Geometry check sheet. Reference: the model listing, model coordinates, mm. Give positions to 0.01 mm unless a question says otherwise; leave off trailing zeros. Write each loop counter-clockwise with the first axis right and the second up, starting at its lowest first coordinate (ties: lowest second). Pieces come first, ordered by that corner, then holes. Notation, with made-up numbers: (73.25, 23.25) - (111.25, 23.25) arc R13 ccw to (111.25, 35.25) - close; hole circle Ø10 at (13, 48.5). An arc over 180 degrees is marked (long way). Use a Markdown table: item, result.
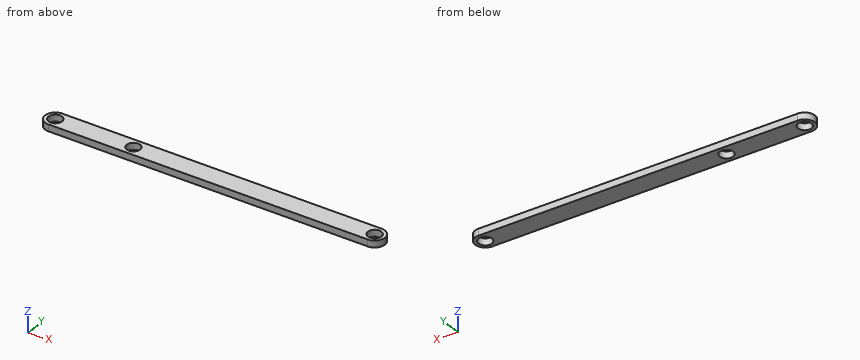
```python
from build123d import *

# Parameters (mm, degrees)
SKETCH3_W           = 250
SKETCH3_H           = 15
BOSS_EXTRUDE4_DEPTH = 5
SKETCH7_R           = 5
CUT_EXTRUDE3_DEPTH  = 5
SKETCH8_R           = 5
CUT_EXTRUDE5_DEPTH  = 6


with BuildPart() as part:
    # Sketch3 → Boss-Extrude4 (new body)
    with BuildSketch(Plane.XY):
        with Locations((-125, 7.5)):
            Rectangle(SKETCH3_W, SKETCH3_H)
    extrude(amount=BOSS_EXTRUDE4_DEPTH)

    # Sketch7 → Cut-Extrude3 (cut)
    with BuildSketch(Plane.XY.offset(5)):
        with BuildLine():
            Line((-242.499999991, 15), (-250, 15))
            Line((-250, 15), (-250, 7.5))
            ThreePointArc((-250, 7.5), (-247.803300856, 12.803300862), (-242.499999991, 15))
        make_face()
        with Locations((-242.5, 7.5)):
            Circle(SKETCH7_R)
        with BuildLine():
            ThreePointArc((-242.5, 0), (-247.803300859, 2.196699141), (-250, 7.5))
            Line((-250, 7.5), (-250, 0))
            Line((-250, 0), (-242.5, 0))
        make_face()
        with BuildLine():
            ThreePointArc((0, 7.5), (-2.196699166, 2.196699116), (-7.50000007, 0))
            Line((-7.50000007, 0), (0, 0))
            Line((0, 0), (0, 7.5))
        make_face()
        with BuildLine():
            Line((0, 15), (-7.5, 15))
            ThreePointArc((-7.5, 15), (-2.196699141, 12.803300859), (0, 7.5))
            Line((0, 7.5), (0, 15))
        make_face()
        with Locations((-7.5, 7.5)):
            Circle(SKETCH7_R)
    extrude(amount=-CUT_EXTRUDE3_DEPTH, mode=Mode.SUBTRACT)

    # Sketch8 → Cut-Extrude5 (cut, through all)
    with BuildSketch(Plane.XY.offset(5)):
        with Locations((-185, 7.5)):
            Circle(SKETCH8_R)
    extrude(amount=-CUT_EXTRUDE5_DEPTH, mode=Mode.SUBTRACT)


solid = part.part
```
1) Section check C-C on x = -185. Record the boundary of the cut face in (y, z), then the cut area to 3 significant figures.
Working result:
| item | result |
|---|---|
| outline | (0, 0) - (2.5, 0) - (2.5, 5) - (0, 5) - close; (12.5, 0) - (15, 0) - (15, 5) - (12.5, 5) - close |
| area | 25.0 mm² |
2) Depth check by flat-ended pin: P1, Ø3, axis at y = 10.5, z = 4.5, coming from the +X side; P2, Ø2, axis at y = 5, z = 1, coming from the -X side; P3, Ø3, axis at y = 1.5, z = 1.5, coming from the +X side. Enter the tip coordinate at first touch or a pass-through.
Working result:
| item | result |
|---|---|
| P1 | stops at x = -0.15 |
| P2 | stops at x = -249.85 |
| P3 | stops at x = -1.5 |
3) Section check A-A on z = 1.15. Record the boundary of the cut face in (x, y), then the cut area to 3 significant figures.
Working result:
| item | result |
|---|---|
| outline | (-242.5, 0) - (-7.5, 0) arc R7.5 ccw to (-7.5, 15) - (-242.5, 15) arc R7.5 ccw to start; hole circle Ø10 at (-242.5, 7.5); hole circle Ø10 at (-185, 7.5); hole circle Ø10 at (-7.5, 7.5) |
| area | 3,470 mm² |
4) Material ranges on L1, parallel to X at y = 4, z = 3.85; L2, parallel to Y at x = -185, z = 1.1; L3, parallel to X at y = 5.5, z = 0.85, recorded low to high. Write a range as from..to.
Working result:
| item | result |
|---|---|
| L1 | x = -249.13..-246.07, -238.93..-188.57, -181.43..-11.07, -3.93..-0.87 |
| L2 | y = 0..2.5, 12.5..15 |
| L3 | x = -249.73..-247.08, -237.92..-189.58, -180.42..-12.08, -2.92..-0.27 |
5) Section check B-B on y = 10. Record the boundary of the cut face in (x, z), then the cut area to 3 significant figures.
Working result:
| item | result |
|---|---|
| outline | (-249.57, 0) - (-246.83, 0) - (-246.83, 5) - (-249.57, 5) - close; (-238.17, 0) - (-189.33, 0) - (-189.33, 5) - (-238.17, 5) - close; (-180.67, 0) - (-11.83, 0) - (-11.83, 5) - (-180.67, 5) - close; (-3.17, 0) - (-0.43, 0) - (-0.43, 5) - (-3.17, 5) - close |
| area | 1,120 mm² |
